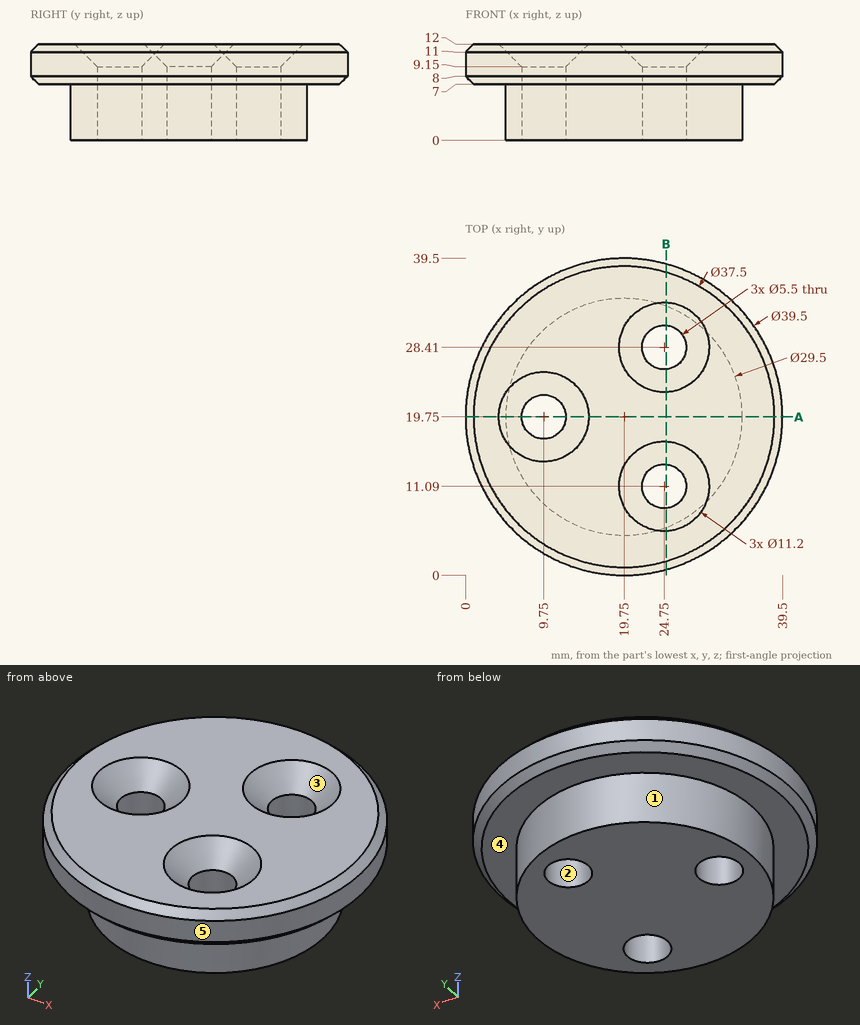
Here's the drawing with two shaded views (mm, measured from the low corner). I have some questions. A direction names the side the tool comes from. Round coordinates to 2 decimals unless told otherwise and drop trailing zeros. Write each loop counter-clockwise with the first axis right and the second up, starting at its lowest first coordinate (ties: lowest second). Pieces come first, ordered by that corner, then holes. Notation, with made-up numbers: M 46,-7.5 L 73,-7.5 A22 ccw 73,27.5 Z; hole C 49,-19.5 d4. An arc over 180 degrees is marked long. Answer in a Markdown table with one row per item. Add a question column.
Q1. Imagine slicing it at A-A (y = 19.75). Please give me the cut outline in (x, z).
Q2. If we mould it in two halves opening along X, with no side actions, what happens to the marked faces 3, 4 and 5? For each: +X half, -X half, draft (parallel to the pull), parting line (faces both ways), or undercut.
Q3. On a 3-axis mill with a long thin cutter (end or side, diameter ignored), from which of +Z, -Z, +X, -X, +Y, -Y can I reach the whole of each face in a straight line? I mean the marked faces 1 and 2. Say none if no direction works.
Q4. Will these pins go through, and if not, where does the flat tip stop? pin 1 Ø3 at (x, z) = (28, 10.5) entering from +Y; pin 2 Ø5 at (y, z) = (17.5, 6.5) entering from -X; pin 3 Ø5 at (y, z) = (19.5, 1.5) entering from +X.
Q5. Imagine slicing it at B-B (x = 25). Give the number of separate pieces and of enclosed holes in the cut face.
Q6. If I drill on line 1 (Y direction, x = 26.5, z = 5.75) (1 decimal); line 2 (Y direction, x = 24.75, z = 4); line 3 (Z direction, x = 22, y = 5), over which ranges is the centre line in solid material (lowest first)? Write a range as from..to.
Values:
| question | item | result |
|---|---|---|
| 1 | outline | M 0,8 L 1,7 L 5,7 L 5,0 L 7,0 L 7,9.15 L 4.15,12 L 1,12 L 0,11 Z; M 12.5,0 L 34.5,0 L 34.5,7 L 38.5,7 L 39.5,8 L 39.5,11 L 38.5,12 L 15.35,12 L 12.5,9.15 Z |
| 2 | face 3 | undercut |
| 2 | face 4 | draft |
| 2 | face 5 | parting line |
| 3 | face 1 | -Z |
| 3 | face 2 | +Z, -Z |
| 4 | pin 1 | y = 38.31 |
| 4 | pin 2 | x = 0 |
| 4 | pin 3 | x = 34.5 |
| 5 | separate pieces | 3 |
| 5 | enclosed holes | 0 |
| 6 | line 1 | 6.6..9, 13.2..26.3, 30.5..32.9 |
| 6 | line 2 | 5.87..8.34, 13.84..25.66, 31.16..33.63 |
| 6 | line 3 | 7..12 |
